Check sheet for the drawn part. Datum: minimum x, y, z corner. Units: mm. A direction names the side the tool comes from. Give positions to 0.01 mm unless a question says otherwise; leave off trailing zeros. Write each loop counter-clockwise with the first axis right and the second up, starting at its lowest first coordinate (ties: lowest second). Pieces come first, ordered by that corner, then holes. Notation, with made-up numbers: (31.25, 88) -> (47.25, 88) arc R19 cw to (47.25, 94) -> close; hole circle Ø2 at (28.25, 14.25). An arc over 180 degrees is marked (long way). Answer as CSV lines item,"result". Start each with the question number.
1) Sectioned sample at D-D on x = 5. Record the cut outline in (y, z), and give its area (3 significant figures).
2) Tool access check on the marked faces 1, 2 and 3. Record the directions out of +Z, -Z, +X, -X, +Y, -Y that give a thin tool (end or side, any length) a straight path to the whole face; none if there is none.
3) Mould release check, pull along Z, two halves, no side actions. Record for the marked faces 4, 5, 6 and 7: released by +Z, released by -Z, zero draft, split by the parting line, or undercut.
4) Material ranges on L1, parallel to Y at x = 4.25, z = 6.75 (1 decimal); L2, parallel to Y at x = 9, z = 11.05; L3, parallel to Z at x = 5.25, y = 4.25 (1 decimal), recorded low to high.
5) Sectioned sample at B-B on z = 11.05. Record the cut outline in (x, y), and give its area (3 significant figures).
6) Sectioned sample at A-A on y = 11.05. Record the cut outline in (x, z) (3 decimals).
7) Gauge pin test, flat ends, axial feed: pin 1 Ø1 at (y, z) = (16.5, 13.5) entering from -X; pin 2 Ø1 at (x, z) = (5.5, 5.5) entering from +Y; pin 3 Ø3 at (y, z) = (18.5, 6) entering from +X; pin 4 Ø2.5 at (y, z) = (5.39, 5.39) entering from +X. Record the tip position at first contact, or that the pin passes through.
8) Sectioned sample at C-C on z = 2.5. Record the cut outline in (x, y) (3 decimals).
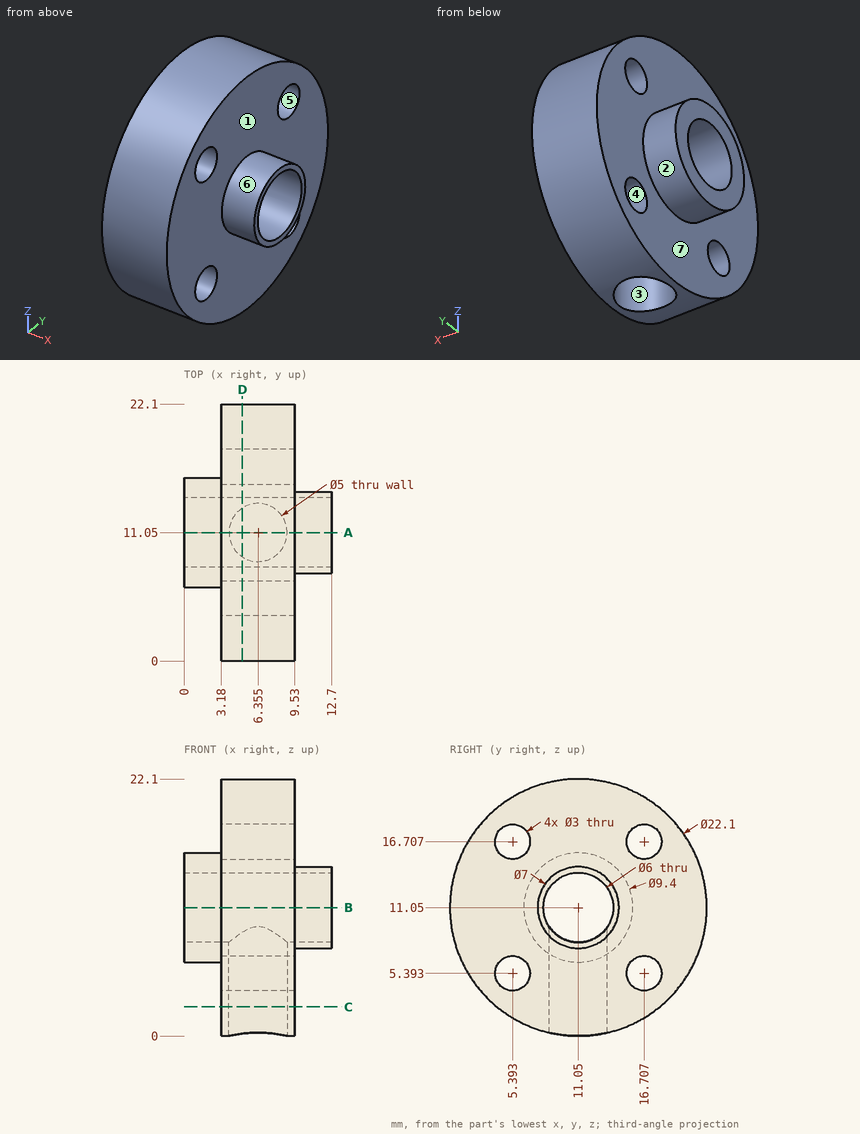
Ans:
1,outline,"(8.95, 0.2) -> (8.95, 8.91) arc R3 cw (long way) to (13.15, 8.91) -> (13.15, 0.2) arc R11.05 ccw (long way) to start; hole circle Ø3 at (5.39, 5.39); hole circle Ø3 at (5.39, 16.71); hole circle Ø3 at (16.71, 5.39); hole circle Ø3 at (16.71, 16.71)"
1,area,"292 mm²"
2,face 1,"+X"
2,face 2,"-X"
2,face 3,"-Z"
3,face 4,"undercut"
3,face 5,"undercut"
3,face 6,"split by the parting line"
3,face 7,"zero draft"
4,L1,"y = 0.9 to 4.8, 6 to 9.7, 12.4 to 16.1, 17.3 to 21.2"
4,L2,"y = 0 to 8.05, 14.05 to 22.1"
4,L3,"z = 2.3 to 4.4, 6.4 to 15.7, 17.7 to 19.8"
5,outline,"(0, 6.35) -> (3.18, 6.35) -> (3.18, 0) -> (9.53, 0) -> (9.53, 7.55) -> (12.7, 7.55) -> (12.7, 8.05) -> (0, 8.05) -> close; (0, 14.05) -> (12.7, 14.05) -> (12.7, 14.55) -> (9.53, 14.55) -> (9.53, 22.1) -> (3.18, 22.1) -> (3.18, 15.75) -> (0, 15.75) -> close"
5,area,"116 mm²"
6,outline,"(0, 6.35) -> (3.18, 6.35) -> (3.18, 0) -> (3.855, 0) -> (3.855, 8.05) -> (0, 8.05) -> close; (0, 14.05) -> (12.7, 14.05) -> (12.7, 14.55) -> (9.53, 14.55) -> (9.53, 22.1) -> (3.18, 22.1) -> (3.18, 15.75) -> (0, 15.75) -> close; (8.855, 0) -> (9.53, 0) -> (9.53, 7.55) -> (12.7, 7.55) -> (12.7, 8.05) -> (8.855, 8.05) -> close"
7,pin 1,"stops at x = 3.18"
7,pin 2,"stops at y = 20.88"
7,pin 3,"stops at x = 9.53"
7,pin 4,"passes through"
8,outline,"(3.18, 4.05) -> (9.53, 4.05) -> (9.53, 18.05) -> (3.18, 18.05) -> close; hole circle Ø5 at (6.355, 11.05)"
